from build123d import *

# Parameters (mm, degrees)
SKETCH1_W           = 175
SKETCH1_H           = 175
BOSS_EXTRUDE1_DEPTH = 15
SKETCH2_W           = 165
SKETCH2_H           = 165
CUT_EXTRUDE1_DEPTH  = 15
SKETCH3_R           = 5
CUT_EXTRUDE2_DEPTH  = 197.230094532


with BuildPart() as part:
    # Sketch1 → Boss-Extrude1 (new body)
    with BuildSketch(Plane(origin=(0, 0, 0), x_dir=(1, 0, 0), z_dir=(0, 1, 0))):
        Rectangle(SKETCH1_W, SKETCH1_H)
    extrude(amount=BOSS_EXTRUDE1_DEPTH)

    # Sketch2 → Cut-Extrude1 (cut)
    with BuildSketch(Plane(origin=(0, 15, 0), x_dir=(1, 0, 0), z_dir=(0, 1, 0))):
        Rectangle(SKETCH2_W, SKETCH2_H)
    extrude(amount=-CUT_EXTRUDE1_DEPTH, mode=Mode.SUBTRACT)

    # Sketch3 → Cut-Extrude2 (cut, through all)
    with BuildSketch(Plane.XY.offset(87.5)):
        with Locations((0, 7.5)):
            Circle(SKETCH3_R)
    extrude(amount=-CUT_EXTRUDE2_DEPTH, mode=Mode.SUBTRACT)


solid = part.part
Geometry check sheet. Reference: the model listing, model coordinates, mm. A direction names the side the tool comes from. Give positions to 0.01 mm unless a question says otherwise; leave off trailing zeros. Write each loop counter-clockwise with the first axis right and the second up, starting at its lowest first coordinate (ties: lowest second). Pieces come first, ordered by that corner, then holes. Notation, with made-up numbers: M -28.5,41 L -11.5,41 A24 ccw -11.5,76 Z; hole C 4,-13 d4. An arc over 180 degrees is marked long. Answer as CSV lines item,"result". Start each with the question number.
Q1. Go/stop test with a flat-tipped pin: pin 1 (9 mm diameter, centred on x = 0, y = 7.5, fed in from +Z). Record where the tip stops, or that it passes through.
Q2. Section check A-A, the plane y = 7.5. Record the cut outline in (x, z).
Q3. Tool access check on faces 1 (the face through (-1, 2, 87.5)), 2 (the face through (-82.5, 8, 1)). Record the directions out of +Z, -Z, +X, -X, +Y, -Y that give a thin tool (end or side, any length) a straight path to the whole face; none if there is none.
Q4. Material ranges on L1, parallel to X at y = 11.75, z = 48.5; L2, parallel to Y at x = 0, z = 84, recorded low to high.
Q5. Section check B-B, the plane z = -10. Record the cut outline in (x, y).
Q6. Section check D-D, the plane x = -48. Record the cut outline in (y, z), then the cut area to 3 significant figures.
Q7. Release check for a two-part mould opening along Z. For faces 3 (the face through (-1, 2, -87.5)), 4 (the face through (-0.651, 12.457, 85.035)), 5 (the face through (-1, 13, 82.5)) record: pulls with the +Z half, pulls with the -Z half, needs draft (parallel to the pull), parting line crosses it, or undercut.
Q8. Section check C-C, the plane x = 0. Record the cut outline in (y, z), then the cut area to 3 significant figures.
Geometry says:
1,pin 1,"through"
2,outline,"M -87.5,-87.5 L -5,-87.5 L -5,-82.5 L -82.5,-82.5 L -82.5,82.5 L -5,82.5 L -5,87.5 L -87.5,87.5 Z; M 5,-87.5 L 87.5,-87.5 L 87.5,87.5 L 5,87.5 L 5,82.5 L 82.5,82.5 L 82.5,-82.5 L 5,-82.5 Z"
3,face 1,"+Z, +X, -X, +Y, -Y"
3,face 2,"+Y, -Y"
4,L1,"-87.5 to -82.5, 82.5 to 87.5"
4,L2,"0 to 2.5, 12.5 to 15"
5,outline,"M -87.5,0 L -82.5,0 L -82.5,15 L -87.5,15 Z; M 82.5,0 L 87.5,0 L 87.5,15 L 82.5,15 Z"
6,outline,"M 0,-87.5 L 15,-87.5 L 15,-82.5 L 0,-82.5 Z; M 0,82.5 L 15,82.5 L 15,87.5 L 0,87.5 Z"
6,area,"150 mm^2"
7,face 3,"pulls with the -Z half"
7,face 4,"needs draft"
7,face 5,"undercut"
8,outline,"M 0,-87.5 L 2.5,-87.5 L 2.5,-82.5 L 0,-82.5 Z; M 0,82.5 L 2.5,82.5 L 2.5,87.5 L 0,87.5 Z; M 12.5,-87.5 L 15,-87.5 L 15,-82.5 L 12.5,-82.5 Z; M 12.5,82.5 L 15,82.5 L 15,87.5 L 12.5,87.5 Z"
8,area,"50.0 mm^2"
